Design review of the part built by this model. Coordinates are the model's own, in mm. A direction names the side the tool comes from. Give positions to 0.01 mm unless a question says otherwise; leave off trailing zeros. Order: outer loops, then holes, each group sorted by start corner. A loop starts at its lowest first (then second) coordinate and runs counter-clockwise, first axis right, second up.
```python
from build123d import *

# Parameters (mm, degrees)
SKETCH_1_R               = 80
SKETCH_1_R_2             = 25
EXTRUDE_1_DEPTH          = 20
EXTRUDE_START            = 15
SKETCH_2_R               = 45
SKETCH_2_R_2             = 25
EXTRUDE_2_DEPTH          = 15
CUT_EXTRUDE_1_DEPTH      = 115.891252931
CUT_EXTRUDE_1_DEPTH_BACK = 115.891252931
SKETCH_3_R               = 7


with BuildPart() as part:
    # 草图1 → 凸台-拉伸1 (new body)
    with BuildSketch(Plane.XY):
        Circle(SKETCH_1_R)
        Circle(SKETCH_1_R_2, mode=Mode.SUBTRACT)
    extrude(amount=-EXTRUDE_1_DEPTH)

    # 草图2 → 凸台-拉伸2 (add)
    with BuildSketch(Plane.XY.offset(EXTRUDE_START)):
        Circle(SKETCH_2_R)
        Circle(SKETCH_2_R_2, mode=Mode.SUBTRACT)
    extrude(amount=-EXTRUDE_2_DEPTH)

    # 草图3 → 切除-拉伸1 (cut, two sides: drawn at the far end of the back side and taken through both)
    with BuildSketch(Plane.XY.offset(-CUT_EXTRUDE_1_DEPTH_BACK)):
        with Locations((62.5, 0)):
            Circle(SKETCH_3_R)
        with Locations((31.25, 54.126587737)):
            Circle(SKETCH_3_R)
        with Locations((-31.25, 54.126587737)):
            Circle(SKETCH_3_R)
        with Locations((-62.5, 0)):
            Circle(SKETCH_3_R)
        with Locations((-31.25, -54.126587737)):
            Circle(SKETCH_3_R)
        with Locations((31.25, -54.126587737)):
            Circle(SKETCH_3_R)
    extrude(amount=CUT_EXTRUDE_1_DEPTH + CUT_EXTRUDE_1_DEPTH_BACK, mode=Mode.SUBTRACT)


solid = part.part
```
1. Draft analysis for pull direction Y (two halves, no side actions). For faces 3 (the face through (-17.34, -78.1, -9.86)), 4 (the face through (-55.823, 2.103, -10.14)), 5 (the face through (34, -34, 0)), 6 (the face through (35.01, 60.03, -10.14)), state which applies: pulls with the +Y half, pulls with the -Y half, needs draft (parallel to the pull), parting line crosses it, or undercut.
Recorded:
face 3: parting line crosses it
face 4: undercut
face 5: needs draft
face 6: undercut
2. For pin 1 (22.5 mm diameter, centred on x = -31.25, y = -54.13, fed in from +Z); pin 2 (11 mm diameter, centred on x = 31.25, y = 54.13, fed in from -Z); pin 3 (10 mm diameter, centred on y = -51, z = -5.5, fed in from +X); pin 4 (4 mm diameter, centred on y = -19.5, z = 8.5, fed in from +X), all flat-tipped, find the tip position at first contact; note any pin that passes through.
Recorded:
pin 1: stops at z = 0
pin 2: passes through
pin 3: stops at x = 65.45
pin 4: stops at x = 41.46
3. Take a section at C-C (z = -17). State the section outline as (x, y) points.
Recorded:
outline: circle Ø160 at (0, 0); hole circle Ø14 at (-62.5, 0); hole circle Ø14 at (-31.25, -54.13); hole circle Ø14 at (-31.25, 54.13); hole circle Ø50 at (0, 0); hole circle Ø14 at (31.25, -54.13); hole circle Ø14 at (31.25, 54.13); hole circle Ø14 at (62.5, 0)
4. Take a section at D-D (y = -57.5). State the section outline as (x, z) points.
Recorded:
outline: (-55.62, -20) - (-37.38, -20) - (-37.38, 0) - (-55.62, 0) - close; (-25.12, -20) - (25.12, -20) - (25.12, 0) - (-25.12, 0) - close; (37.38, -20) - (55.62, -20) - (55.62, 0) - (37.38, 0) - close
5. Take a section at B-B (x = 31.25). State the section outline as (y, z) points, then the cut area to 3 significant figures.
Recorded:
outline: (-73.64, -20) - (-61.13, -20) - (-61.13, 0) - (-73.64, 0) - close; (-47.13, -20) - (47.13, -20) - (47.13, 0) - (32.38, 0) - (32.38, 15) - (-32.38, 15) - (-32.38, 0) - (-47.13, 0) - close; (61.13, -20) - (73.64, -20) - (73.64, 0) - (61.13, 0) - close
area: 3,360 mm2
6. Machinability: for faces 1 (the face through (69.177, 2.103, -10.14)), 2 (the face through (20.765, -39.923, 7.605)), which of the approach directions +Z, -Z, +X, -X, +Y, -Y give a long, thin tool a straight path to every point of the face, cutting with its end or side? Answer none if there is none.
Recorded:
face 1: +Z, -Z
face 2: +Z
7. Take a section at A-A (x = 0). State the section outline as (y, z) points.
Recorded:
outline: (-80, -20) - (-25, -20) - (-25, 15) - (-45, 15) - (-45, 0) - (-80, 0) - close; (25, -20) - (80, -20) - (80, 0) - (45, 0) - (45, 15) - (25, 15) - close
8. For line 1 along Y through (x, z) = (-29, -4); line 2 along X through (y, z) = (-1, -6); line 3 along Y through (x, z) = (-31.25, -6.75), list the stretches that pass through material, from the lowest coordinate up.
Recorded:
line 1: y = -74.56 to -60.76, -47.5 to 47.5, 60.76 to 74.56
line 2: x = -79.99 to -69.43, -55.57 to -24.98, 24.98 to 55.57, 69.43 to 79.99
line 3: y = -73.64 to -61.13, -47.13 to 47.13, 61.13 to 73.64
